Build history of the part. All positions in model axes, mm. A direction names the side the tool comes from. Round coordinates to 2 decimals unless told otherwise and drop trailing zeros. Loops run counter-clockwise (first coordinate to the right, second up) from the corner with the lowest first, then second, coordinate; pieces in that order, holes last. Notation, with made-up numbers: (-17.75, -18.75) - (9.25, -18.75) arc R27 ccw to (9.25, 0.25) - close; hole circle Ø1 at (38, 28). An arc over 180 degrees is marked (long way). Use one line per item in the form item = value. Start each with the question number.
Q1. Saw through at A-A (z = 18). Give the cut face in (x, y) (1 decimal), then the cut area to 3 significant figures.
Q2. Pin check, flat tips, straight feed: pin 1 (3 mm diameter, centred on x = 6.5, z = 22.5, fed in from +Y) (3 decimals); pin 2 (5.5 mm diameter, centred on y = 20, z = 32.5, fed in from -X); pin 3 (12 mm diameter, centred on y = 35, z = 27.5, fed in from -X). Stop position of each tip, or through.
Q3. Saw through at C-C (y = 42). Give the cut face in (x, z).
Q4. Mould opens along X. For faces 6 (the face through (-53.93, -25.44, 12.32)), 7 (the face through (5, 64.425, 17)), 8 (the face through (10, 62, 16)) say: released by +X, released by -X, zero draft, split by the parting line, or undercut.
Q5. Saw through at D-D (x = 5). Give the cut face in (y, z) (3 decimals), then the cut area to 3 significant figures.
Q6. 3-axis set-ups, long thin cutter, end or side, ignore diameter. For faces 1 (the face through (-52.24, -30.16, 23.54)), 2 (the face through (53.33, -36.48, 17.33)), 3 (the face through (49, -33.98, 12.32)), 4 (the face through (21.469, -12.395, 32.535)), 5 (the face through (-16.955, 63.277, 2.465)): which of +Z, -Z, +X, -X, +Y, -Y reach the whole face in a straight line?
Q7. Drill centre lines: line 1 (Y direction, x = 5, z = 32); line 2 (Y direction, x = 0.5, z = 6) (3 decimals); line 3 (Y direction, x = -22.5, z = 32). Where is each one in solid material? Low to high.
Q8. Saw through at B-B (x = -30.5). Give the cut face in (y, z).
Autodesk Inventor part; units mm, degrees
ref_plane "YZ Plane" through (0, 0, 0) normal (1, 0, 0) x (0, 1, 0)
ref_plane "XZ Plane" through (0, 0, 0) normal (0, 1, 0) x (-1, 0, 0)
ref_plane "XY Plane" through (0, 0, 0) normal (0, 0, 1) x (1, 0, 0)
sketch "Sketch1" plane through (0, 0, 0) normal (0, 0, 1) x (1, 0, 0)
  circle A0 centre (0, 0) radius 59.425
  circle A1 centre (0, 0) radius 71.425
  line L0 (0, 0) -> (0, 59.425) construction
  line L1 (0, 71.425) -> (0, 59.425) construction
  circle A2 centre (0, 0) radius 65.075
  dimension "d0" = 118.85
  dimension "d2" = 12
  dimension "d12" = 130.15
sketch "Sketch2" plane through (0, 0, 0) normal (1, 0, 0) x (0, 1, 0)
  line L0 (59.425, 0) -> (59.425, 25)
  line L1 (54.425, 30) -> (0, 30)
  line L2 (59.425, 35) -> (0, 35)
  line L3 (0, 35) -> (0, 30)
  line L4 (71.425, 0) -> (71.425, 5)
  line L5 (71.425, 5) -> (64.425, 5)
  line L6 (64.425, 5) -> (64.425, 30)
  arc A0 (64.425, 30) -> (59.425, 35) centre (59.425, 30) ccw
  arc A1 (59.425, 25) -> (54.425, 30) centre (54.425, 25) ccw
  line L7 (71.425, 0) -> (59.425, 0)
  point P0 (0, 0)
  dimension "d3" = 5
  dimension "d5" = 30
  dimension "d6" = 5
  dimension "d7" = 5
  dimension "d8" = 5
extrude "Extrusion2" add sketch "Sketch2" along normal blind 10
sketch "Sketch5" plane through (0, 0, 0) normal (-1, 0, 0) x (0, 0, 1)
  line L0 (5, 71.425) -> (0, 71.425)
  line L1 (0, 71.425) -> (0, 59.425)
  line L2 (0, 59.425) -> (5, 59.425)
  line L3 (5, 59.425) -> (5, 71.425)
  line L4 (-7, 0) -> (42, 0)
  point P0 (0, 0)
revolve "Revolution1" add sketch "Sketch5" angle 15 about axis through (0, 0, -10) along (0, 0, 1)
sketch "Sketch6" plane through (0, 64.425, 5) normal (0, 0, 1) x (1, 0, 0)
  circle A0 centre (0, -64.425) radius 65.075 construction
  circle A1 centre (-8.494, 0.0933) radius 4
  line L0 (-8.494, 0.0933) -> (0, 7) construction
  line L1 (-18.4862, 4.5663) -> (-8.494, 0.0933) construction
  dimension "d17" = 8
extrude "Extrusion3" cut sketch "Sketch6" against normal blind 10
pattern_circular "Circular Pattern1" count 3 over 360 about axis through (0, 0, -10) along (0, 0, 1) of "Extrusion2", "Revolution1", "Extrusion3"
sketch "Sketch7" plane through (0, 59.425, 35) normal (0, 0, 1) x (1, 0, 0)
  circle A0 centre (0, -59.425) radius 50
  circle A1 centre (0, -59.425) radius 40
  circle A2 centre (0, -59.425) radius 65.075
  circle A3 centre (0, -59.425) radius 10
  point P0 (-5, -50.7647)
  dimension "d23" = 100
  dimension "d24" = 80
extrude "Extrusion4" add sketch "Sketch7" against normal blind 5 contours A0 | A3
sketch "Sketch8" plane through (0, 59.425, 35) normal (0, 0, 1) x (1, 0, 0)
  circle A0 centre (5, -14.425) radius 6.25
  line L0 (0, -19.425) -> (0, -49.425)
  circle A1 centre (5, -14.425) radius 12.25
  circle A2 centre (-2.7942, -9.925) radius 1.5
  circle A3 centre (5, -23.425) radius 1.5
  circle A4 centre (12.7942, -9.925) radius 1.5
  circle A5 centre (5, -14.425) radius 9 construction
  line L1 (5, -23.425) -> (-2.7942, -9.925) construction
  line L2 (12.7942, -9.925) -> (-2.7942, -9.925) construction
  line L3 (5, -23.425) -> (12.7942, -9.925) construction
  point P0 (0, -59.425)
  dimension "d27" = 12.5
  dimension "d28" = 5
  dimension "d29" = 45
  dimension "d32" = 6
  dimension "d35" = 3
  dimension "d36" = 3
  dimension "d37" = 3
  dimension "d38" = 18
extrude "Extrusion6" add sketch "Sketch8" against normal blind 5 contours A1 | A2 | A3 | A4
extrude "Extrusion5" cut sketch "Sketch8" against normal blind 5 contours A0 | A2 | A3 | A4
properties part number "Return_Spool_Mount_2"
Report:
q1.outline = (-60.8, -23.6) - (-55.8, -32.2) - (-51.5, -29.7) - (-56.5, -21.1) - close; (0, 59.4) - (10, 59.4) - (10, 64.4) - (0, 64.4) - close; (46.5, -38.4) - (50.8, -40.9) - (55.8, -32.2) - (51.5, -29.7) - close
q1.area = 150 mm²
q2.pin_1 = 64.425
q2.pin_2 = -46.93
q2.pin_3 = -40.34
q3.outline = (-27.13, 30) - (-0.48, 30) - (-0.48, 35) - (-27.13, 35) - close; (10.48, 30) - (27.13, 30) - (27.13, 35) - (10.48, 35) - close
q4.face_6 = undercut
q4.face_7 = zero draft
q4.face_8 = released by +X
q5.outline = (-49.749, 30) - (-39.686, 30) - (-39.686, 35) - (-49.749, 35) - close; (-14.434, 30) - (34.5, 30) - (34.5, 35) - (-14.434, 35) - close; (37.5, 30) - (38.75, 30) - (38.75, 35) - (37.5, 35) - close; (51.25, 30) - (54.425, 30) arc R5 cw to (59.425, 25) - (59.425, 0) - (71.425, 0) - (71.425, 5) - (64.425, 5) - (64.425, 30) arc R5 ccw to (59.425, 35) - (51.25, 35) - close
q5.area = 552 mm²
q6.face_1 = +Z, -Y
q6.face_2 = +Z, +X, -Y
q6.face_3 = -Z, +Y
q6.face_4 = +Z, -Z
q6.face_5 = +Z, -Z, -X, -Y
q7.line_1 = -49.75 to -39.69, -14.43 to 34.5, 37.5 to 38.75, 51.25 to 64.01
q7.line_2 = 59.425 to 64.425
q7.line_3 = -44.65 to -33.07, -12.99 to -1.44, 33.07 to 44.65
q8.outline = (-39.62, 30) - (-25.88, 30) - (-25.88, 35) - (-39.62, 35) - close; (-17.61, 30) - (-6.06, 30) - (-6.06, 35) - (-17.61, 35) - close; (25.88, 30) - (39.62, 30) - (39.62, 35) - (25.88, 35) - close
